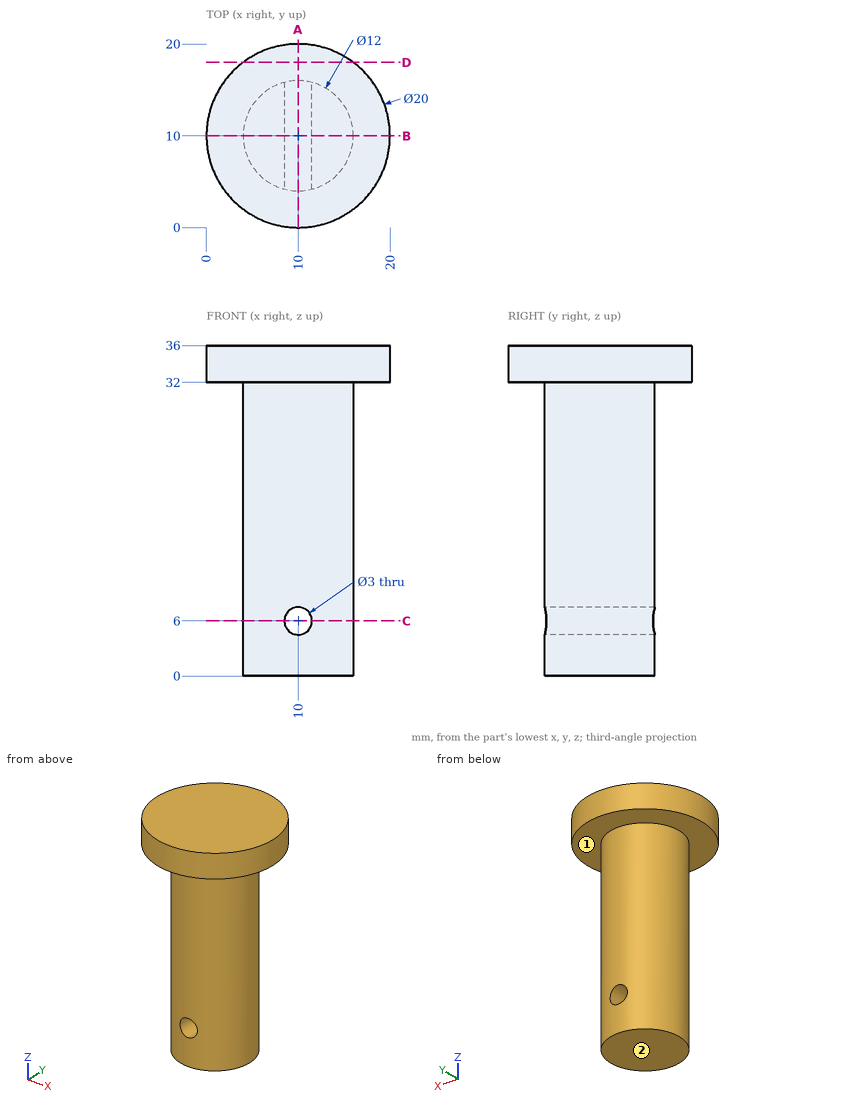
Check sheet for the drawn part. Datum: minimum x, y, z corner. Units: mm. A direction names the side the tool comes from. Coordinates: 2 decimals unless noted, no trailing zeros. Order: outer loops, then holes, each group sorted by start corner. A loop starts at its lowest first (then second) coordinate and runs counter-clockwise, first axis right, second up. Notation, with made-up numbers: M -35.75,20.25 L -13.75,20.25 A20 cw -13.75,53.25 Z; hole C -36.75,31.25 d2. An arc over 180 degrees is marked long. One line per item, written item: value. Start each with the question number.
Item 1: Access from +Z, -Z, +X, -X, +Y, -Y to the whole of each face (thin tool, end or side, straight path). Record for the marked faces 1 and 2.
Item 2: Sectioned sample at B-B (y = 10). Enter the section's corners in (x, z), then the cut area to 3 significant figures.
Item 3: Sectioned sample at D-D (y = 18). Enter the section's corners in (x, z), then the cut area to 3 significant figures.
Item 4: Sectioned sample at A-A (x = 10). Enter the section's corners in (y, z).
Item 5: Sectioned sample at C-C (z = 6). Enter the section's corners in (x, y).
Item 6: Gauge pin test, flat ends, axial feed: pin 1 (4 mm diameter, centred on x = 10, z = 6, fed in from +Y); pin 2 (3 mm diameter, centred on y = 9.5, z = 5.5, fed in from +X); pin 3 (1.5 mm diameter, centred on x = 15, y = 2, fed in from -Z). Record the tip position at first contact, or that the pin passes through.
Item 7: Scan lines: probe 1 along Z at (x, y) = (10, 7.25); probe 2 along Z at (x, y) = (14, 17.75); probe 3 along X at (y, z) = (5.5, 6.5). Record each from-to range of solid material in increasing order.
Conclusion:
1. face 1: -Z
1. face 2: -Z, +X, -X, +Y, -Y
2. outline: M 0,32 L 4,32 L 4,0 L 16,0 L 16,32 L 20,32 L 20,36 L 0,36 Z; hole C 10,6 d3
2. area: 457 mm^2
3. outline: M 4,32 L 16,32 L 16,36 L 4,36 Z
3. area: 48.0 mm^2
4. outline: M 0,32 L 4,32 L 4,7.5 L 16,7.5 L 16,32 L 20,32 L 20,36 L 0,36 Z; M 4,0 L 16,0 L 16,4.5 L 4,4.5 Z
5. outline: M 8.5,4.19 L 8.5,15.81 A6 ccw Z; M 11.5,4.19 A6 ccw 11.5,15.81 Z
6. pin 1: stops at y = 16
6. pin 2: stops at x = 16
6. pin 3: stops at z = 32
7. probe 1: z = 0 to 4.5, 7.5 to 36
7. probe 2: z = 32 to 36
7. probe 3: x = 6.03 to 8.59, 11.41 to 13.97
